Geometry: final body of the model. Coordinates: model frame, mm. Face numbers are marked on the shaded views. A direction names the side the tool comes from. Give positions to 0.01 mm unless a question says otherwise; leave off trailing zeros. Write each loop counter-clockwise with the first axis right and the second up, starting at its lowest first coordinate (ties: lowest second). Pieces come first, ordered by that corner, then holes. Notation, with made-up numbers: M -38.75,5 L 9.25,5 A18 ccw 9.25,22 Z; hole C 58.25,78 d11. An arc over 180 degrees is marked long. Use one line per item in the form item = value. Start each with the question number.
Item 1: Section query A-A on x = -8.5. Return loops of the section in (y, z), then the cut area to 3 significant figures.
Item 2: Section query C-C on y = 7.5. Return loops of the section in (x, z), then the cut area to 3 significant figures.
Item 3: Material intervals for line 1 along X through (y, z) = (15.75, -73.5); line 2 along Z through (x, y) = (-23, 3.25); line 3 along Y through (x, z) = (4, -132), sorted ascending. Write a range as from..to.
Item 4: Section query B-B on z = 6.5. Return loops of the section in (x, y), then the cut area to 3 significant figures.
Item 5: Access query for the marked faces 4 and 5. Directions: +Z, -Z, +X, -X, +Y, -Y. A direction counts if a zero-diameter tool reaches every point of the face in a straight line with its end or side. Return the directions, or none.
Item 6: Pull-direction query (Z, two-part tool) for the marked faces 1, 2 and 3; classes: released by +Z, released by -Z, zero draft, split by the parting line, or undercut.
Item 7: Contact query for flat-ended pins moving along their axis: P1, Ø4, axis at x = 2.5, y = 5, coming from the +Z side; P2, Ø3, axis at x = 4.27, z = -151.38, coming from the +Y side; P3, Ø3, axis at x = -23.5, z = -152, coming from the +Y side; P4, Ø1, axis at x = -32, y = 14, coming from the -Z side. Output: stop coordinate, or through.
Autodesk Inventor part; units mm, degrees
ref_plane "YZ Plane" through (0, 0, 0) normal (1, 0, 0) x (0, 1, 0)
ref_plane "XZ Plane" through (0, 0, 0) normal (0, 1, 0) x (-1, 0, 0)
ref_plane "XY Plane" through (0, 0, 0) normal (0, 0, 1) x (1, 0, 0)
sketch "Sketch1" plane through (0, 0, 0) normal (0, 1, 0) x (-1, 0, 0)
  line L0 (40.5829, -68.5109) -> (-9.4171, -68.5109)
  line L1 (-9.4171, -68.5109) -> (-9.4171, 7.9891)
  line L2 (-9.4171, 7.9891) -> (40.5829, 7.9891)
  line L3 (40.5829, 7.9891) -> (40.5829, -68.5109)
  line L4 (40.5829, -68.5109) -> (-9.4171, -68.5109)
  line L5 (-9.4171, -68.5109) -> (-9.4171, -145.0109)
  line L6 (-9.4171, -145.0109) -> (40.5829, -145.0109)
  line L7 (40.5829, -145.0109) -> (40.5829, -68.5109)
  line L8 (43.2164, 17.8584) -> (43.2164, -154.8803)
  line L9 (43.2164, -68.5109) -> (-11.5522, -68.5109)
  line L10 (-11.5522, -68.5109) -> (-11.5522, -147.7105)
  line L11 (-11.5522, -147.7105) -> (43.2164, -147.7105)
  line L12 (43.2164, -147.7105) -> (43.2164, -68.5109)
  line L13 (-11.5522, 10.6887) -> (43.2164, 10.6887)
  line L14 (-11.5522, -68.5109) -> (-11.5522, 10.6887)
  circle A0 centre (-4.2663, -151.3765) radius 1.65
  circle A1 centre (32.2203, -151.3765) radius 1.65
  line L15 (43.2164, -147.7105) -> (43.2164, -154.8803)
  line L16 (43.2164, -154.8803) -> (-11.5522, -154.8803)
  line L17 (-13.2912, -151.8803) -> (16.3367, -151.8803)
  line L18 (-11.5522, -154.8803) -> (-11.5522, -147.7105)
  line L19 (-11.5522, 10.6887) -> (43.2164, 10.6887)
  line L20 (-13.2912, 14.8584) -> (16.3367, 14.8584)
  circle A2 centre (-4.2663, 14.3547) radius 1.65
  line L21 (-11.5522, 17.8584) -> (-11.5522, 10.6887)
  line L22 (43.2164, 17.8584) -> (-11.5522, 17.8584)
  circle A3 centre (32.2203, 14.3547) radius 1.65
  line L23 (43.2164, 10.6887) -> (43.2164, 17.8584)
  point P0 (0, 0)
  point P1 (7.1317, -61.1506)
  point P2 (-9.4171, -68.5109)
  dimension "d2" = 50
  dimension "d3" = 76.5
  dimension "d4" = 76.5
  dimension "d5" = 3.3
  dimension "d6" = 3.3
extrude "Extrusion1" add sketch "Sketch1" along normal blind 18 contours L9 L8 L11 L10 L5 L6 L7 | L3 L2 L1 L9 L14 L13 L8
extrude "Extrusion2" add sketch "Sketch1" along normal blind 2 contours L7 L6 L5 L0 | L0 L1 L2 L3 | L13 L21 L22 L8 | L8 L16 L18 L11
fillet "Fillet1" radius 1.5 1 edges at (-15.8321, 2, -147.7105)
fillet "Fillet2" radius 1.5 1 edges at (-15.8321, 2, 10.6887)
properties part number "beban"
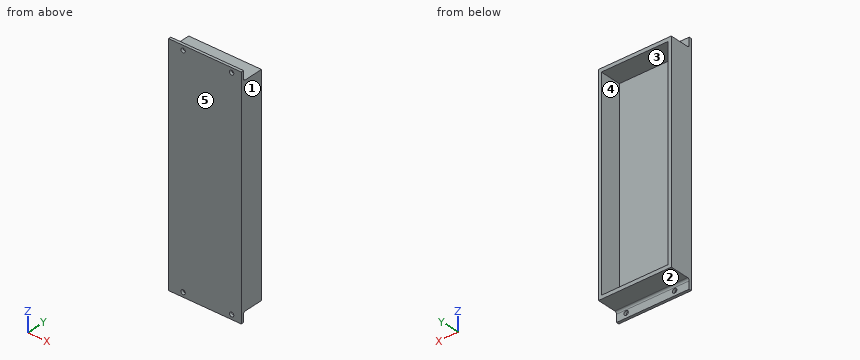
Answer sheet:
q1.outline = M 0,-154.88 L 2,-154.88 L 2,-149.21 A1.5 cw 3.5,-147.71 L 18,-147.71 L 18,-145.01 L 2,-145.01 L 2,7.99 L 18,7.99 L 18,10.69 L 3.5,10.69 A1.5 cw 2,12.19 L 2,17.86 L 0,17.86 Z
q1.area = 433 mm2
q2.outline = M -43.22,-147.71 L 11.55,-147.71 L 11.55,10.69 L -43.22,10.69 Z; hole M -40.58,-145.01 L 9.42,-145.01 L 9.42,7.99 L -40.58,7.99 Z
q2.area = 1,030 mm2
q3.line_1 = -43.22..-40.58, 9.42..11.55
q3.line_2 = -147.73..-145.01, 7.99..10.71
q3.line_3 = 0..2
q4.outline = M -43.22,0 L 11.55,0 L 11.55,18 L 9.42,18 L 9.42,2 L -40.58,2 L -40.58,18 L -43.22,18 Z
q4.area = 186 mm2
q5.face_4 = +Y
q5.face_5 = +Z, -Z, +X, -X, -Y
q6.face_1 = zero draft
q6.face_2 = released by -Z
q6.face_3 = undercut
q7.P1 = 10.77
q7.P2 = through
q7.P3 = 2
q7.P4 = -147.71
